from build123d import *

# Parameters (mm, degrees)
SKETCH1_R           = 2.75
BOSS_EXTRUDE1_DEPTH = 3.2
SKETCH2_R           = 1.4
BOSS_EXTRUDE2_DEPTH = 8.3
BOSS_EXTRUDE3_DEPTH = 4.2


with BuildPart() as part:
    # Sketch1 → Boss-Extrude1 (new body)
    with BuildSketch(Plane(origin=(0, 0, 0), x_dir=(1, 0, 0), z_dir=(0, 1, 0))):
        Circle(SKETCH1_R)
    extrude(amount=BOSS_EXTRUDE1_DEPTH)

    # Sketch2 → Boss-Extrude2 (add)
    with BuildSketch(Plane(origin=(0, 3.2, 0), x_dir=(1, 0, 0), z_dir=(0, 1, 0))):
        Circle(SKETCH2_R)
    extrude(amount=BOSS_EXTRUDE2_DEPTH)

    # Sketch3 → Boss-Extrude3 (add)
    with BuildSketch(Plane(origin=(0, 11.5, 0), x_dir=(1, 0, 0), z_dir=(0, 1, 0))):
        Polygon((1.554649618, 2.702418281), (-1.563038074, 2.697575204), (-3.117687692, -0.004843077), (-1.554649618, -2.702418281), (1.563038074, -2.697575204), (3.117687692, 0.004843077), align=None)
    extrude(amount=BOSS_EXTRUDE3_DEPTH)


solid = part.part
Input: part model. Units: mm. Frame: model coordinates. A direction names the side the tool comes from. Round coordinates to 2 decimals unless told otherwise and drop trailing zeros. Write each loop counter-clockwise with the first axis right and the second up, starting at its lowest first coordinate (ties: lowest second). Pieces come first, ordered by that corner, then holes.
1) Cut plane B-B (x = 0). Return the cut outline in (y, z), then the cut area to 3 significant figures.
2) Reachability of faces 1 (the cylindrical face through (-1.4, 7.29, -0.06)), 2 (the flat face through (2.329, 13.571, 1.365)), 3 (the cylindrical face through (-0.596, 1.578, 2.685)) from +Z, -Z, +X, -X, +Y, -Y: full face, straight path, thin tool, end or side. Return the list, or none.
3) Cut plane D-D (z = 0.5). Return the cut outline in (x, y), then the cut area to 3 significant figures.
4) Ray query, L1, parallel to Y at x = 2.5, z = 0.3; L2, parallel to Z at x = -0.75, y = 15; L3, parallel to Z at x = -1, y = 2. Return the intervals inside material, ascending.
5) Cut plane C-C (y = 5.75). Return the cut outline in (x, z).
6) Cut plane A-A (z = -2.15). Return the cut outline in (x, y), then the cut area to 3 significant figures.
7) Contact query for flat-ended pins moving along their axis: P1, Ø1, axis at x = 0, y = 4, coming from the +Z side; P2, Ø1.5, axis at x = 1.5, y = 12, coming from the -Z side; P3, Ø3, axis at y = 13, z = -2, coming from the +X side. Output: stop coordinate, or through.
Geometry says:
1. outline: (0, -2.75) - (3.2, -2.75) - (3.2, -1.4) - (11.5, -1.4) - (11.5, -2.7) - (15.7, -2.7) - (15.7, 2.7) - (11.5, 2.7) - (11.5, 1.4) - (3.2, 1.4) - (3.2, 2.75) - (0, 2.75) - close
1. area: 63.5 mm2
2. face 1: none
2. face 2: +Z, +X, +Y
2. face 3: -Y
3. outline: (-2.83, 11.5) - (-1.31, 11.5) - (-1.31, 3.2) - (-2.7, 3.2) - (-2.7, 0) - (2.7, 0) - (2.7, 3.2) - (1.31, 3.2) - (1.31, 11.5) - (2.83, 11.5) - (2.83, 15.7) - (-2.83, 15.7) - close
3. area: 62.8 mm2
4. L1: y = 0 to 3.2, 11.5 to 15.7
4. L2: z = -2.7 to 2.7
4. L3: z = -2.56 to 2.56
5. outline: circle Ø2.8 at (0, 0)
6. outline: (-1.88, 11.5) - (1.87, 11.5) - (1.87, 15.7) - (-1.88, 15.7) - close; (-1.71, 0) - (1.71, 0) - (1.71, 3.2) - (-1.71, 3.2) - close
6. area: 26.7 mm2
7. P1: stops at z = 1.4
7. P2: stops at z = -2.7
7. P3: stops at x = 2.83
